Read the model definition and answer for the solid it produces. Units are mm, in the model's axes. Coordinates: 2 decimals unless noted, no trailing zeros. Loops run counter-clockwise (first coordinate to the right, second up) from the corner with the lowest first, then second, coordinate; pieces in that order, holes last.
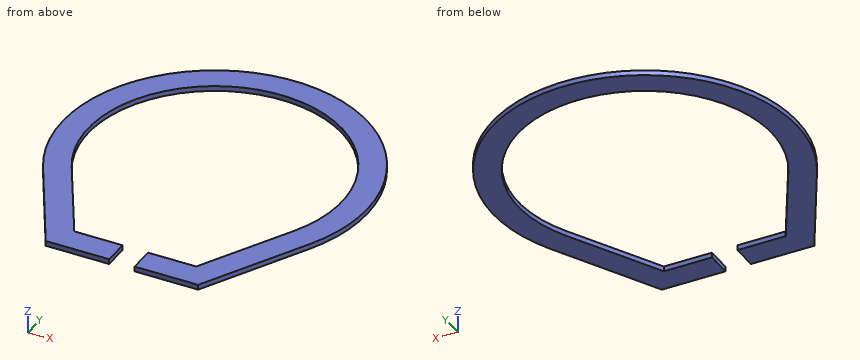
from build123d import *

# Parameters (mm, degrees)
RESSALTO_EXTRUS_O3_DEPTH = 1


with BuildPart() as part:
    # Esboço1 → Ressalto-extrusão3 (new body)
    with BuildSketch(Plane.XY):
        with BuildLine():
            Line((5, -35), (15, -35))
            Line((15, -35), (26.292884648, -14.44590658))
            ThreePointArc((26.292884648, -14.44590658), (0, 30), (-26.292884648, -14.44590658))
            Line((-26.292884648, -14.44590658), (-15, -35))
            Line((-15, -35), (-5, -35))
            Line((-5, -35), (-2.5, -35))
            Line((-2.5, -35), (-2.5, -32.5))
            Line((-2.5, -32.5), (-2.5, -30))
            Line((-2.5, -30), (-5, -30))
            Line((-5, -30), (-12, -30))
            Line((-12, -30), (-21.889001071, -12.077732905))
            ThreePointArc((-21.889001071, -12.077732905), (0, 25), (21.889001071, -12.077732905))
            Line((21.889001071, -12.077732905), (12, -30))
            Line((12, -30), (5, -30))
            Line((5, -30), (2.5, -30))
            Line((2.5, -30), (2.5, -32.5))
            Line((2.5, -32.5), (2.5, -35))
            Line((2.5, -35), (5, -35))
        make_face()
    extrude(amount=RESSALTO_EXTRUS_O3_DEPTH)


solid = part.part
Item 1: A cutting plane is placed at D-D on x = 0. Determine the outline of the cut face in (y, z).
Numbers:
outline: (25, 0) - (30, 0) - (30, 1) - (25, 1) - close
Item 2: A cutting plane is placed at B-B on x = 6.5. Determine the outline of the cut face in (y, z).
Numbers:
outline: (-35, 0) - (-30, 0) - (-30, 1) - (-35, 1) - close; (24.14, 0) - (29.29, 0) - (29.29, 1) - (24.14, 1) - close
Item 3: A cutting plane is placed at C-C on z = 0.2. Determine the outline of the cut face in (x, y), then the cut area to 3 significant figures.
Numbers:
outline: (-26.29, -14.45) - (-15, -35) - (-2.5, -35) - (-2.5, -30) - (-12, -30) - (-21.89, -12.08) arc R25 cw (long way) to (21.89, -12.08) - (12, -30) - (2.5, -30) - (2.5, -35) - (15, -35) - (26.29, -14.45) arc R30 ccw (long way) to start
area: 901 mm2
Item 4: Find the intervals of material crossed by line 1 along X through (y, z) = (0, 0.8); line 2 along Y through (x, z) = (22, 0.5); line 3 along Y through (x, z) = (15, 0.2), in increasing order.
Numbers:
line 1: x = -30 to -25, 25 to 30
line 2: y = -22.26 to -11.87, 11.87 to 20.4
line 3: y = -35 to -24.56, 20 to 25.98
Item 5: Given pin 1 (1 mm diameter, centred on x = 22.5, y = 1.5, fed in from -Z), flat-ended and moving along its own axis, determine where the tip first touches the part or whether it passes through.
Numbers:
pin 1: passes through
Item 6: A cutting plane is placed at A-A on y = 0. Determine the outline of the cut face in (x, z).
Numbers:
outline: (-30, 0) - (-25, 0) - (-25, 1) - (-30, 1) - close; (25, 0) - (30, 0) - (30, 1) - (25, 1) - close
